from build123d import *

# Parameters (mm, degrees)
SKETCH11_W                                     = 160
SKETCH11_H                                     = 60
SKETCH11_R                                     = 2.55
SKETCH11_R_2                                   = 6
BOSS_EXTRUDE1_DEPTH                            = 3
FILLET1_R                                      = 2
FILLET3_R                                      = 3
CSK_FOR_M3_FLAT_HEAD_MACHINE_SCREW1_AT_2_COUNT = 2
CSK_FOR_M3_FLAT_HEAD_MACHINE_SCREW1_AT_2_PITCH = 22.042551394
CSK_FOR_M3_FLAT_HEAD_MACHINE_SCREW1_AT_3_COUNT = 2
CSK_FOR_M3_FLAT_HEAD_MACHINE_SCREW1_AT_3_PITCH = 45
CSK_FOR_M3_FLAT_HEAD_MACHINE_SCREW1_AT_4_COUNT = 2
CSK_FOR_M3_FLAT_HEAD_MACHINE_SCREW1_AT_4_PITCH = 137.493516675
CSK_FOR_M3_FLAT_HEAD_MACHINE_SCREW1_AT_5_COUNT = 2
CSK_FOR_M3_FLAT_HEAD_MACHINE_SCREW1_AT_5_PITCH = 131.893933603
CSK_FOR_M3_FLAT_HEAD_MACHINE_SCREW1_AT_6_COUNT = 2
CSK_FOR_M3_FLAT_HEAD_MACHINE_SCREW1_AT_6_PITCH = 130.000201211
CSK_FOR_M3_FLAT_HEAD_MACHINE_SCREW1_AT_7_COUNT = 2
CSK_FOR_M3_FLAT_HEAD_MACHINE_SCREW1_AT_7_PITCH = 65.174880681
CSK_FOR_M3_FLAT_HEAD_MACHINE_SCREW1_AT_8_COUNT = 2
CSK_FOR_M3_FLAT_HEAD_MACHINE_SCREW1_AT_8_PITCH = 76.202062771


with BuildPart() as part:
    # Sketch11 → Boss-Extrude1 (new body)
    with BuildSketch(Plane.XY):
        with Locations((-80, 30)):
            Rectangle(SKETCH11_W, SKETCH11_H)
        with Locations((-35, 50)):
            Circle(SKETCH11_R, mode=Mode.SUBTRACT)
        with Locations((-55, 45)):
            Circle(SKETCH11_R_2, mode=Mode.SUBTRACT)
        with BuildLine():
            Line((-44.886859967, 31.5), (-45.897247359, 31.5))
            Line((-45.897247359, 31.5), (-45.897247359, 28.5))
            Line((-45.897247359, 28.5), (-44.886859967, 28.5))
            ThreePointArc((-44.886859967, 28.5), (-42.370691635, 23.241826814), (-37.35, 20.280046296))
            Line((-37.35, 20.280046296), (-37.35, 19.253954216))
            Line((-37.35, 19.253954216), (-32.65, 19.253954216))
            Line((-32.65, 19.253954216), (-32.65, 20.280046296))
            ThreePointArc((-32.65, 20.280046296), (-27.629308365, 23.241826814), (-25.113140033, 28.5))
            Line((-25.113140033, 28.5), (-24.102752641, 28.5))
            Line((-24.102752641, 28.5), (-24.102752641, 31.5))
            Line((-24.102752641, 31.5), (-25.113140033, 31.5))
            ThreePointArc((-25.113140033, 31.5), (-27.629308365, 36.758173186), (-32.65, 39.719953704))
            Line((-32.65, 39.719953704), (-32.65, 40.746045784))
            Line((-32.65, 40.746045784), (-37.35, 40.746045784))
            Line((-37.35, 40.746045784), (-37.35, 39.719953704))
            ThreePointArc((-37.35, 39.719953704), (-42.370691635, 36.758173186), (-44.886859967, 31.5))
        make_face(mode=Mode.SUBTRACT)
        with BuildLine():
            Line((-83.627304882, 41.930328357), (-77.227304882, 41.930328357))
            ThreePointArc((-77.227304882, 41.930328357), (-71.227304882, 35.930328357), (-77.227304882, 29.930328357))
            Line((-77.227304882, 29.930328357), (-83.627304882, 29.930328357))
            ThreePointArc((-83.627304882, 29.930328357), (-89.627304882, 35.930328357), (-83.627304882, 41.930328357))
        make_face(mode=Mode.SUBTRACT)
        with BuildLine():
            Line((-110.715747539, 41.9), (-104.315747539, 41.9))
            ThreePointArc((-104.315747539, 41.9), (-98.315747539, 35.9), (-104.315747539, 29.9))
            Line((-104.315747539, 29.9), (-110.715747539, 29.9))
            ThreePointArc((-110.715747539, 29.9), (-116.715747539, 35.9), (-110.715747539, 41.9))
        make_face(mode=Mode.SUBTRACT)
    extrude(amount=BOSS_EXTRUDE1_DEPTH)

    # Fillet1
    fillet1_edges = [part.edges().sort_by_distance(p)[0] for p in [
        (-160, 30, 3),
        (-80, 0, 3),
        (0, 30, 3),
    ]]
    fillet(fillet1_edges, radius=FILLET1_R)

    # Fillet3
    # the kernel refuses this fillet: 3 mm, written as the material it takes off along each edge
    with BuildSketch(Plane(origin=(-3, 3, 3), x_dir=(0, -1, 0), z_dir=(-1, 0, 0))) as fillet3_piece_1:
        with BuildLine():
            CenterArc((1, -2), 2, 0, 90)
            Line((3, -2), (3, 0))
            Line((3, 0), (1, 0))
        make_face()
    revolve(axis=Axis((-3, 3, 3), (0, 0, 1)), revolution_arc=90, mode=Mode.SUBTRACT)
    with BuildSketch(Plane(origin=(-157, 3, 3), x_dir=(-1, 0, 0), z_dir=(0, 1, 0))) as fillet3_piece_2:
        with BuildLine():
            CenterArc((1, -2), 2, 0, 90)
            Line((3, -2), (3, 0))
            Line((3, 0), (1, 0))
        make_face()
    revolve(axis=Axis((-157, 3, 3), (0, 0, 1)), revolution_arc=90, mode=Mode.SUBTRACT)
    with BuildSketch(Plane(origin=(0, 0, -7.5), x_dir=(-1, 0, 0), z_dir=(0, 0, 1))) as fillet3_piece_3:
        with BuildLine():
            CenterArc((FILLET3_R, -FILLET3_R), FILLET3_R, 90, 90)
            Line((0, -FILLET3_R), (0, 0))
            Line((0, 0), (FILLET3_R, 0))
        make_face()
    extrude(amount=10.5, mode=Mode.SUBTRACT)
    with BuildSketch(Plane(origin=(-160, 0, -7.5), x_dir=(1, 0, 0), z_dir=(0, 0, 1))) as fillet3_piece_4:
        with BuildLine():
            CenterArc((FILLET3_R, FILLET3_R), FILLET3_R, 180, 90)
            Line((0, FILLET3_R), (0, 0))
            Line((0, 0), (FILLET3_R, 0))
        make_face()
    extrude(amount=10.5, mode=Mode.SUBTRACT)

    # Sketch13 → CSK for M3 Flat Head Machine Screw1 (revolve, cut)
    with BuildSketch(Plane(origin=(-145, 54.771275697, 3), x_dir=(0, -1, 0), z_dir=(1, 0, 0))):
        Polygon((0, 0), (0, 3), (1.7, 3), (1.7, 1.45), (3.15, 0), align=None)
    csk_for_m3_flat_head_machine_screw1 = revolve(axis=Axis((-145, 54.771275697, 9.35), (0, 0, -1)), mode=Mode.SUBTRACT)

    # CSK for M3 Flat Head Machine Screw1 at 2: CSK for M3 Flat Head Machine Screw1 ×2
    with Locations(*[(0, -i * CSK_FOR_M3_FLAT_HEAD_MACHINE_SCREW1_AT_2_PITCH, 0) for i in range(1, CSK_FOR_M3_FLAT_HEAD_MACHINE_SCREW1_AT_2_COUNT)]):
        add(csk_for_m3_flat_head_machine_screw1, mode=Mode.SUBTRACT)

    # CSK for M3 Flat Head Machine Screw1 at 3: CSK for M3 Flat Head Machine Screw1 ×2
    with Locations(*[(0, -i * CSK_FOR_M3_FLAT_HEAD_MACHINE_SCREW1_AT_3_PITCH, 0) for i in range(1, CSK_FOR_M3_FLAT_HEAD_MACHINE_SCREW1_AT_3_COUNT)]):
        add(csk_for_m3_flat_head_machine_screw1, mode=Mode.SUBTRACT)

    # CSK for M3 Flat Head Machine Screw1 at 4: CSK for M3 Flat Head Machine Screw1 ×2
    with Locations(*[Vector(0.9454991271168814, -0.32562463147190707, 0) * (i * CSK_FOR_M3_FLAT_HEAD_MACHINE_SCREW1_AT_4_PITCH) for i in range(1, CSK_FOR_M3_FLAT_HEAD_MACHINE_SCREW1_AT_4_COUNT)]):
        add(csk_for_m3_flat_head_machine_screw1, mode=Mode.SUBTRACT)

    # CSK for M3 Flat Head Machine Screw1 at 5: CSK for M3 Flat Head Machine Screw1 ×2
    with Locations(*[Vector(0.9856404798092461, -0.16885746818367017, 0) * (i * CSK_FOR_M3_FLAT_HEAD_MACHINE_SCREW1_AT_5_PITCH) for i in range(1, CSK_FOR_M3_FLAT_HEAD_MACHINE_SCREW1_AT_5_COUNT)]):
        add(csk_for_m3_flat_head_machine_screw1, mode=Mode.SUBTRACT)

    # CSK for M3 Flat Head Machine Screw1 at 6: CSK for M3 Flat Head Machine Screw1 ×2
    with Locations(*[Vector(0.9999984522282437, 0.001759414992816724, 0) * (i * CSK_FOR_M3_FLAT_HEAD_MACHINE_SCREW1_AT_6_PITCH) for i in range(1, CSK_FOR_M3_FLAT_HEAD_MACHINE_SCREW1_AT_6_COUNT)]):
        add(csk_for_m3_flat_head_machine_screw1, mode=Mode.SUBTRACT)

    # CSK for M3 Flat Head Machine Screw1 at 7: CSK for M3 Flat Head Machine Screw1 ×2
    with Locations(*[Vector(0.997316747201951, -0.07320727935472046, 0) * (i * CSK_FOR_M3_FLAT_HEAD_MACHINE_SCREW1_AT_7_PITCH) for i in range(1, CSK_FOR_M3_FLAT_HEAD_MACHINE_SCREW1_AT_7_COUNT)]):
        add(csk_for_m3_flat_head_machine_screw1, mode=Mode.SUBTRACT)

    # CSK for M3 Flat Head Machine Screw1 at 8: CSK for M3 Flat Head Machine Screw1 ×2
    with Locations(*[Vector(0.8529952817065795, -0.5219186233373103, 0) * (i * CSK_FOR_M3_FLAT_HEAD_MACHINE_SCREW1_AT_8_PITCH) for i in range(1, CSK_FOR_M3_FLAT_HEAD_MACHINE_SCREW1_AT_8_COUNT)]):
        add(csk_for_m3_flat_head_machine_screw1, mode=Mode.SUBTRACT)


solid = part.part
Can you work these out from the model? Positions are in its coordinate system, mm. Coordinates: 2 decimals unless noted, no trailing zeros. Write each loop counter-clockwise with the first axis right and the second up, starting at its lowest first coordinate (ties: lowest second). Pieces come first, ordered by that corner, then holes. Notation, with made-up numbers: M 87,-9 L 136,-9 A7 cw 136,-1 Z; hole C 80,71 d3. An arc over 180 degrees is marked long. Use one line per item in the form item = value.
Q1. If we section it at A-A (y = 15): Write out the boundary of the cut face in (x, z), then the cut area to 3 significant figures.
Model answer:
outline = M -160,0 L -81.7,0 L -81.7,1.55 L -83.15,3 L -158,3 A2 ccw -160,1 Z; M -78.3,0 L 0,0 L 0,1 A2 ccw -2,3 L -76.85,3 L -78.3,1.55 Z
area = 466 mm^2
Q2. We'd pull the mould along Y, two halves only. Please class faces 1 (the flat face through (-107, 29.9, 1)), 2 (the flat face through (-80, 29.93, 1)): +Y half, -Y half, draft (parallel to the pull), parting line (faces both ways), or undercut.
Model answer:
face_1 = undercut
face_2 = undercut
Q3. If we section it at B-B (x = -55): Write out the boundary of the cut face in (y, z), then the cut area to 3 significant figures.
Model answer:
outline = M 0,0 L 39,0 L 39,3 L 2,3 A2 ccw 0,1 Z; M 51,0 L 60,0 L 60,3 L 51,3 Z
area = 143 mm^2
Q4. For P1, Ø1, axis at y = 6, z = 2.5, coming from the -X side; P2, Ø0.8, axis at y = 19.5, z = 1.5, coming from the -X side; P3, Ø0.8, axis at y = 40, z = 1.5, coming from the +X side, each with a flat end and sliding along its axis, tell me the tip position at first contact or that it passes through.
Model answer:
P1 = -159.73
P2 = -160
P3 = 0
Q5. If we section it at D-D (x = -28.5): Write out the boundary of the cut face in (y, z).
Model answer:
outline = M 0,0 L 22.4,0 L 22.4,3 L 2,3 A2 ccw 0,1 Z; M 37.6,0 L 60,0 L 60,3 L 37.6,3 Z
Q6. I need wall thicknesses on line 1 along Y through (x, z) = (-145, 0.6); line 2 along Y through (x, z) = (-35, 1.1); line 3 along X through (y, z) = (15, 0.95). Which ranges of each line are inside material? Lowest first, please. Write a range as from..to.
Model answer:
line_1 = 0..8.07, 11.47..31.03, 34.43..53.07, 56.47..60
line_2 = 0..19.25, 40.75..47.45, 52.55..60
line_3 = -160..-81.7, -78.3..0
Q7. If we section it at C-C (y = 55): State how many separate pieces and enclosed holes the cut face has, then the cut area to 3 significant figures.
Model answer:
separate_pieces = 3
enclosed_holes = 0
area = 454 mm^2
